Design review of the part built by this model. Coordinates are the model's own, in mm. A direction names the side the tool comes from. Coordinates: 2 decimals unless noted, no trailing zeros. Write each loop counter-clockwise with the first axis right and the second up, starting at its lowest first coordinate (ties: lowest second). Pieces come first, ordered by that corner, then holes. Notation, with made-up numbers: (-29.75, 32.25) - (22.25, 32.25) arc R13 ccw to (22.25, 37.25) - close; hole circle Ø2 at (58.5, -40). An arc over 180 degrees is marked (long way). Use a Markdown table: item, result.
Autodesk Inventor part; units mm, degrees
ref_plane "YZ Plane" through (0, 0, 0) normal (1, 0, 0) x (0, 1, 0)
ref_plane "XZ Plane" through (0, 0, 0) normal (0, 1, 0) x (-1, 0, 0)
ref_plane "XY Plane" through (0, 0, 0) normal (0, 0, 1) x (1, 0, 0)
sketch "Skizze1" plane through (0, 0, 0) normal (0, 0, 1) x (1, 0, 0)
  line L0 (0, 0) -> (-35, 0)
  line L1 (-35, 0) -> (-35, 35)
  line L2 (-35, 35) -> (0, 35)
  line L3 (0, 35) -> (0, 0)
  dimension "d0" = 35
  dimension "d1" = 35
extrude "NEMA11 Halter" add sketch "Skizze1" along normal blind 6
sketch "Skizze2" plane through (0, 0, 6) normal (0, 0, 1) x (1, 0, 0)
  circle A0 centre (-17.5, 17.5) radius 12.5
  dimension "d4" = 25
extrude "Motorloch" cut sketch "Skizze2" against normal up to surface (6 mm away)
sketch "Skizze3" plane through (0, 0, 6) normal (0, 0, 1) x (1, 0, 0)
  circle A0 centre (-29, 29) radius 1.4
  circle A1 centre (-17.5, 17.5) radius 12.5
  line L0 (-35, 0) -> (-35, 35)
  line L1 (0, 0) -> (-35, 0)
  line L2 (0, 35) -> (0, 0)
  line L3 (-35, 35) -> (0, 35)
  circle A2 centre (-6, 29) radius 1.4
  circle A3 centre (-29, 6) radius 1.4
  circle A4 centre (-6, 6) radius 1.4
  dimension "d7" = 2.8
  dimension "d8" = 2.8
  dimension "d9" = 23
  dimension "d10" = 2.8
  dimension "d11" = 23
  dimension "d12" = 2.8
  dimension "d13" = 23
  dimension "d14" = 23
extrude "Motorschrauben" cut sketch "Skizze3" against normal up to surface (6 mm away) contours A0 | A2 | A3 | A4
sketch "Skizze22" plane through (0, 0, 6) normal (0, 0, 1) x (1, 0, 0)
  circle A0 centre (-6, 6) radius 1.4
  circle A1 centre (-29, 29) radius 1.4
  circle A2 centre (-6, 29) radius 1.4
  circle A3 centre (-29, 6) radius 1.4
  circle A4 centre (-29, 29) radius 2.5
  circle A5 centre (-6, 29) radius 2.5
  circle A6 centre (-6, 6) radius 2.5
  circle A7 centre (-29, 6) radius 2.5
  dimension "d78" = 5
  dimension "d79" = 5
  dimension "d80" = 5
  dimension "d81" = 5
extrude "Extrusion16" cut sketch "Skizze22" against normal blind 1
sketch "Skizze23" plane through (0, 0, 6) normal (0, 0, 1) x (1, 0, 0)
  line L0 (0, 35) -> (100, 35)
  line L1 (100, 35) -> (100, 0)
  line L2 (100, 0) -> (0, 0)
  line L3 (0, 0) -> (0, 35)
  dimension "d84" = 100
extrude "Extrusion17" add sketch "Skizze23" against normal blind 6
sketch "Skizze24" plane through (-35, 0, 0) normal (0, -1, 0) x (1, 0, 0)
  line L0 (135, 0) -> (141, 0)
  line L1 (141, 0) -> (141, 55)
  line L2 (141, 55) -> (135, 55)
  line L3 (135, 55) -> (135, 0)
  point P0 (35, 0)
  dimension "d87" = 6
  dimension "d88" = 55
extrude "Extrusion18" add sketch "Skizze24" against normal up to surface (35 mm away)
fillet "Rundung8" radius 5 1 edges at (100, 17.5, 6)
fillet "Rundung9" radius 1 2 edges at (103, 0, 55) (103, 35, 55)
fillet "Rundung10" radius 1 2 edges at (-35, 0, 3) (-35, 35, 3)
sketch "Skizze25" plane through (100, 0, 11) normal (-1, 0, 0) x (0, 0, 1)
  circle A0 centre (36.6571, 29.1388) radius 1.5
  circle A1 centre (36.6571, 6.8732) radius 1.5
  circle A2 centre (11.524, 29.1388) radius 1.5
  circle A3 centre (11.524, 6.8732) radius 1.5
  point P0 (-11, 0)
  dimension "d94" = 3
  dimension "d95" = 3
  dimension "d96" = 3
  dimension "d97" = 3
extrude "Extrusion19" cut sketch "Skizze25" against normal up to surface (6 mm away)
properties part number "Einfach Nema"
(1) Take a section at D-D on x = 52. Write out the cut boundary in (y, z).
Determined:
| item | result |
|---|---|
| outline | (0, 0) - (35, 0) - (35, 6) - (0, 6) - close |
(2) Take a section at B-B on x = -17.5. Write out the cut boundary in (y, z).
Determined:
| item | result |
|---|---|
| outline | (0, 0) - (5, 0) - (5, 6) - (0, 6) - close; (30, 0) - (35, 0) - (35, 6) - (30, 6) - close |
(3) For L1, parallel to X at y = 17, z = 1; L2, parallel to Y at x = -29, z = 1.85; L3, parallel to X at y = 18, z = 22.5, list the stretches that pass through material, from the lowest coordinate up. Write a range as from..to.
Determined:
| item | result |
|---|---|
| L1 | -35..-29.99, -5.01..106 |
| L2 | 0..4.6, 7.4..12.6, 22.4..27.6, 30.4..35 |
| L3 | 100..106 |
(4) For pin 1 (5.5 mm diameter, centred on x = -6.5, y = 5, fed in from +Z); pin 2 (4 mm diameter, centred on y = 29.14, z = 22.52, fed in from -X); pin 3 (2.5 mm diameter, centred on x = -6, y = 29, fed in from +Z); pin 4 (1.5 mm diameter, centred on x = -29.5, y = 28, fed in from +Z), all flat-tipped, find the tip position at first contact; note any pin that passes through.
Determined:
| item | result |
|---|---|
| pin 1 | z = 6 |
| pin 2 | x = 100 |
| pin 3 | through |
| pin 4 | z = 5 |
(5) Draft analysis for pull direction Z (two halves, no side actions). For faces 4 (the flat face through (-27.9, 4.9, 5)), 5 (the cylindrical face through (102.958, 5.96, 46.467)), 6 (the cylindrical face through (-29.33, 31.48, 5.51)), state which applies: +Z half, -Z half, draft (parallel to the pull), parting line (faces both ways), or undercut.
Determined:
| item | result |
|---|---|
| face 4 | +Z half |
| face 5 | undercut |
| face 6 | draft |
(6) Machinability: for faces 1 (the flat face through (106, 17, 27)), 2 (the cylindrical face through (-3.615, 6.751, 5.507)), 3 (the flat face through (44, 18, 6)), which of the approach directions +Z, -Z, +X, -X, +Y, -Y give a long, thin tool a straight path to every point of the face, cutting with its end or side? Answer none if there is none.
Determined:
| item | result |
|---|---|
| face 1 | +Z, -Z, +X, +Y, -Y |
| face 2 | +Z |
| face 3 | +Z, -X, +Y, -Y |
(7) Take a section at C-C on z = 18. Write out the cut boundary in (x, y), and give its area (3 significant figures).
Determined:
| item | result |
|---|---|
| outline | (100, 0) - (106, 0) - (106, 35) - (100, 35) - close |
| area | 210 mm2 |
(8) Take a section at A-A on y = 14. Write out the cut boundary in (x, z).
Determined:
| item | result |
|---|---|
| outline | (-35, 0) - (-29.5, 0) - (-29.5, 6) - (-35, 6) - close; (-5.5, 0) - (106, 0) - (106, 55) - (100, 55) - (100, 11) arc R5 cw to (95, 6) - (-5.5, 6) - close |
